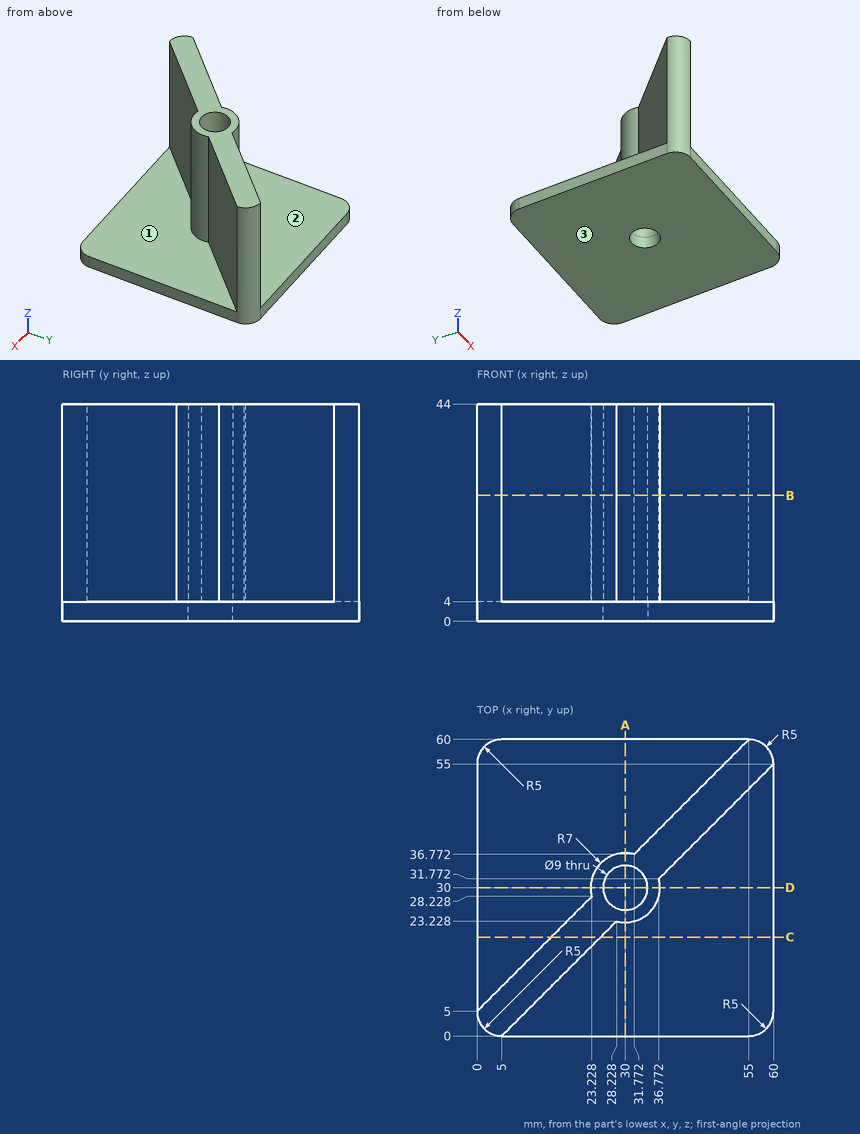
Verification items for this drawing (mm, ordinates from the low corner). A direction names the side the tool comes from. Give positions to 0.01 mm unless a question says otherwise; leave off trailing zeros. Loops run counter-clockwise (first coordinate to the right, second up) from the corner with the lowest first, then second, coordinate; pieces in that order, holes last. Notation, with made-up numbers: (-24, 24) - (24, 24) arc R7 ccw to (24, 35) - close; hole circle Ø3 at (37, 6). An arc over 180 degrees is marked (long way). Write item = value, one per line. Start each with the question number.
Q1. Cross-section at B-B, the plane z = 25.5. Enter the section's corners in (x, y).
Q2. Thickness scan on line 1 (Y direction, x = 30, z = 36.5); line 2 (Y direction, x = 30, z = 1); line 3 (Z direction, x = 38.5, y = 11.5). Record the ranges inside material, lowest first.
Q3. Depth check by flat-ended pin: P1, Ø14.5, axis at x = 30, y = 30, coming from the -Z side; P2, Ø10, axis at x = 46, z = 18, coming from the -Y side; P3, Ø12, axis at y = 47.5, z = 27.5, coming from the +X side; P4, Ø2, axis at y = 34, z = 14, coming from the -X side. Enter the tip coordinate at first touch or a pass-through.
Q4. Cross-section at C-C, the plane y = 20. Enter the section's corners in (x, z), and give its area (3 significant figures).
Q5. Tool access check on the marked faces 1, 2 and 3. Record the directions out of +Z, -Z, +X, -X, +Y, -Y that give a thin tool (end or side, any length) a straight path to the whole face; none if there is none.
Q6. Cross-section at A-A, the plane x = 30. Enter the section's corners in (y, z), and give its area (3 significant figures).
Answer key:
q1.outline = (0, 5) arc R5 ccw to (5, 0) - (28.23, 23.23) arc R7 ccw to (36.77, 31.77) - (60, 55) arc R5 ccw to (55, 60) - (31.77, 36.77) arc R7 ccw to (23.23, 28.23) - close; hole circle Ø9 at (30, 30)
q2.line_1 = 23 to 25.5, 34.5 to 37
q2.line_2 = 0 to 25.5, 34.5 to 60
q2.line_3 = 0 to 4
q3.P1 = 0
q3.P2 = 36
q3.P3 = 58.5
q3.P4 = 23.68
q4.outline = (0, 0) - (60, 0) - (60, 4) - (25, 4) - (25, 44) - (15, 44) - (15, 4) - (0, 4) - close
q4.area = 640 mm^2
q5.face_1 = +Z, +X, -Y
q5.face_2 = +Z, -X, +Y
q5.face_3 = -Z, +X, -X, +Y, -Y
q6.outline = (0, 0) - (25.5, 0) - (25.5, 44) - (23, 44) - (23, 4) - (0, 4) - close; (34.5, 0) - (60, 0) - (60, 4) - (37, 4) - (37, 44) - (34.5, 44) - close
q6.area = 404 mm^2
